Check sheet for the modelled part. Datum: model origin and axes. Units: mm. A direction names the side the tool comes from. Give positions to 0.01 mm unless a question says otherwise; leave off trailing zeros. Loops run counter-clockwise (first coordinate to the right, second up) from the corner with the lowest first, then second, coordinate; pieces in that order, holes last. Notation, with made-up numbers: (73.5, -36) - (88.5, -36) arc R36 cw to (88.5, -2) - close; hole circle Ø11 at (-38, 17.5). An arc over 180 degrees is marked (long way). Use CSV: the item, a comma, the result in double quotes.
from build123d import *

# Parameters (mm, degrees)
F0_R     = 209.55
F1_DEPTH = 19.05
F2_R     = 171.45
F3_DEPTH = 25.4
F4_R     = 207.9625
F4_R_2   = 198.4375
F5_DEPTH = 19.05


with BuildPart() as f1:
    # F0 (on Top) → F1 (new body)
    with BuildSketch(Plane.XY):
        Circle(F0_R)
    extrude(amount=F1_DEPTH)

    # F2 (on face) → F3 (cut)
    with BuildSketch(Plane(origin=(0, 0, 0), x_dir=(1, 0, 0), z_dir=(0, 0, -1))):
        Circle(F2_R)
    extrude(amount=-F3_DEPTH, mode=Mode.SUBTRACT)

    # F4 (on face) → F5 (join)
    with BuildSketch(Plane.XY.offset(19.05)):
        Circle(F4_R)
        Circle(F4_R_2, mode=Mode.SUBTRACT)
    extrude(amount=F5_DEPTH)


solid = f1.part
1. Sectioned sample at A-A, the plane x = 0. Record the boundary of the cut face in (y, z).
Completed:
outline,"(-209.55, 0) - (-171.45, 0) - (-171.45, 19.05) - (-198.44, 19.05) - (-198.44, 38.1) - (-207.96, 38.1) - (-207.96, 19.05) - (-209.55, 19.05) - close; (171.45, 0) - (209.55, 0) - (209.55, 19.05) - (207.96, 19.05) - (207.96, 38.1) - (198.44, 38.1) - (198.44, 19.05) - (171.45, 19.05) - close"
2. Sectioned sample at C-C, the plane z = 13. Record the boundary of the cut face in (x, y).
Completed:
outline,"circle Ø419.1 at (0, 0); hole circle Ø342.9 at (0, 0)"
3. Set-up check for faces 4 (the face through (-43.02, -193.72, 28.44)), 5 (the face through (-172, 1, 0)): record each of +Z, -Z, +X, -X, +Y, -Y from which the full face is reachable in a straight line by a thin tool's end or side.
Completed:
face 4,"+Z"
face 5,"-Z, +X, -X, +Y, -Y"
4. Release check for a two-part mould opening along Y. For faces 1 (the face through (184, -76, 38.1)), 2 (the face through (92.17, -144.567, 9.392)), 3 (the face through (-45.082, -203.017, 28.442)) record: released by +Y, released by -Y, zero draft, split by the parting line, or undercut.
Completed:
face 1,"zero draft"
face 2,"undercut"
face 3,"split by the parting line"
5. Go/stop test with flat-tipped pins: pin 1 Ø1 at (y, z) = (99, 27.5) entering from -X; pin 2 Ø1 at (x, z) = (-138, 29) entering from +Y; pin 3 Ø6 at (x, z) = (-64.5, 29.5) entering from +Y. Record where each tip stops, or that it passes through.
Completed:
pin 1,"stops at x = -183.16"
pin 2,"stops at y = 156.02"
pin 3,"stops at y = 198.66"
6. Scan lines: line 1 along Y through (x, z) = (0, 33); line 2 along Y through (x, z) = (0, 4); line 3 along Z through (x, y) = (-181, -73.5). Record each from-to range of solid material in increasing order.
Completed:
line 1,"y = -207.96 to -198.44, 198.44 to 207.96"
line 2,"y = -209.55 to -171.45, 171.45 to 209.55"
line 3,"z = 0 to 19.05"
